Work out the finished part from the listing and answer in its coordinate system (mm). Face numbers are marked on the shaded views. A direction names the side the tool comes from. Coordinates: 2 decimals unless noted, no trailing zeros. Order: outer loops, then holes, each group sorted by start corner. A loop starts at its lowest first (then second) coordinate and runs counter-clockwise, first axis right, second up. Notation, with made-up numbers: (73, -8) -> (87, -8) arc R21 cw to (87, -1) -> close; hole circle Ø9 at (33, 66). An arc over 180 degrees is marked (long way). Write item = value, one per line. Start each with the question number.
Q1. Straight lines are drawn through the part: L1, parallel to Y at x = -243.2, z = 60; L2, parallel to Y at x = -25, z = 9.1; L3, parallel to X at y = -5.75, z = 85.5. For each, find the intervals that lie inside material, in ascending order. Write a range as from..to.
Q2. The part is cut by section C-C, the plane z = 60. Determine the outline of the cut face in (x, y).
Q3. The part is cut by section B-B, the plane x = -233. Determine the outline of the cut face in (y, z).
Q4. The part is cut by section D-D, the plane x = -49. Determine the outline of the cut face in (y, z).
Q5. Which of the six approach directions +Z, -Z, +X, -X, +Y, -Y give full straight-line access (tool end or side, diameter ignored) to the marked faces 1 and 2?
Q6. The part is cut by section A-A, the plane z = 104.5. Determine the outline of the cut face in (x, y), plus the area to 3 significant figures.
Q7. Flat-ended cylindrical pins translate along their axes: pin 1 (10 mm diameter, centred on y = 3, z = 135, fed in from +X); pin 2 (8 mm diameter, centred on y = 7, z = 112.5, fed in from +X); pin 3 (12.5 mm diameter, centred on x = -78.5, y = -3, fed in from +Z); pin 4 (15 mm diameter, centred on y = 3.5, z = 94, fed in from -X). Find the tip coordinate at first contact, or state that the pin passes through.
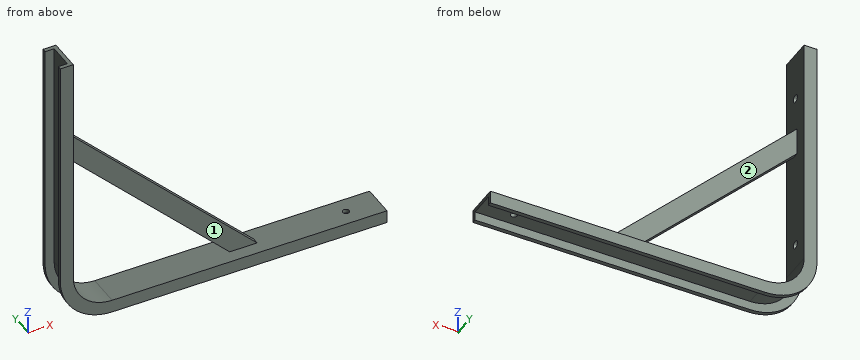
```python
from build123d import *

# Parameters (mm, degrees)
ESQUISSE1_W                  = 450
ESQUISSE1_H                  = 25
EXTRUSION1_DEPTH             = 10
PLIAGE_START                 = -12.5
PLIAGE_1_DEPTH               = 25
PLIAGE_1_2_DEPTH             = 25
ESQUISSE5_R                  = 3
ENL_V_MAT_EXTRU_1_DEPTH      = 330.361564282
ESQUISSE7_R                  = 2.5
ENL_V_MAT_EXTRU_2_DEPTH      = 331.27116136
ENL_V_MAT_EXTRU_3_DEPTH      = 9.5
ENL_V_MAT_EXTRU_3_DEPTH_BACK = 9.5
EXTRUSION2_DEPTH             = 2.5


# Read off the part's stored shape, not the designer's step: Pliage 1
with BuildPart() as part:
    # Esquisse1 → Extrusion1 (new body)
    with BuildSketch(Plane.XY):
        with Locations((-225, 0)):
            Rectangle(ESQUISSE1_W, ESQUISSE1_H)
    extrude(amount=EXTRUSION1_DEPTH)

    # Pliage 1 outline → Pliage 1 (cut)
    with BuildSketch(Plane(origin=(0, 0, 0), x_dir=(1, 0, 0), z_dir=(0, 1, 0)).offset(PLIAGE_START)):
        with BuildLine():
            Line((-450, -10), (-238.968577392, -10))
            ThreePointArc((-238.968577392, -10), (-226.653199905, -2.583426132), (-212.511064281, 0))
            Line((-212.511064281, 0), (-450, 0))
            Line((-450, 0), (-450, -10))
        make_face()
    extrude(amount=PLIAGE_1_DEPTH, mode=Mode.SUBTRACT)

    # Pliage 1 2 outline → Pliage 1 2 (add)
    with BuildSketch(Plane(origin=(0, 0, 0), x_dir=(1, 0, 0), z_dir=(0, 1, 0)).offset(PLIAGE_START)):
        with BuildLine():
            ThreePointArc((-238.968577392, -10), (-248.968577392, -23.542486889), (-252.511064281, -40))
            Line((-252.511064281, -40), (-252.511064281, -222.511064281))
            Line((-252.511064281, -222.511064281), (-242.511064281, -222.511064281))
            Line((-242.511064281, -222.511064281), (-242.511064281, -40))
            ThreePointArc((-242.511064281, -40), (-233.724267717, -18.786796564), (-212.511064281, -10))
            Line((-212.511064281, -10), (-238.968577392, -10))
        make_face()
    extrude(amount=PLIAGE_1_2_DEPTH)

    # Esquisse5 → Enlèv. mat.-Extru.1 (cut, through all)
    with BuildSketch(Plane(origin=(-242.511064281, 0, 0), x_dir=(0, 0, -1), z_dir=(1, 0, 0))):
        with Locations((-185, 0)):
            Circle(ESQUISSE5_R)
        with Locations((-60, 0)):
            Circle(ESQUISSE5_R)
    extrude(amount=-ENL_V_MAT_EXTRU_1_DEPTH, mode=Mode.SUBTRACT)

    # Esquisse7 → Enlèv. mat.-Extru.2 (cut, through all)
    with BuildSketch(Plane.XY.offset(10)):
        with Locations((-25, 0)):
            Circle(ESQUISSE7_R)
    extrude(amount=-ENL_V_MAT_EXTRU_2_DEPTH, mode=Mode.SUBTRACT)

    # Esquisse8 → Enlèv. mat.-Extru.3 (cut, two sides: drawn at the far end of the back side and taken through both)
    with BuildSketch(Plane(origin=(0, 0, 0), x_dir=(1, 0, 0), z_dir=(0, 1, 0)).offset(-ENL_V_MAT_EXTRU_3_DEPTH_BACK)):
        with BuildLine():
            Line((0, -7), (-212.511064281, -7))
            ThreePointArc((-212.511064281, -7), (-235.84558806, -16.665476221), (-245.511064281, -40))
            Line((-245.511064281, -40), (-245.511064281, -222.511064281))
            Line((-245.511064281, -222.511064281), (-252.511064281, -222.511064281))
            Line((-252.511064281, -222.511064281), (-252.511064281, -40))
            ThreePointArc((-252.511064281, -40), (-240.795335529, -11.715728753), (-212.511064281, 0))
            Line((-212.511064281, 0), (0, 0))
            Line((0, 0), (0, -7))
        make_face()
    extrude(amount=ENL_V_MAT_EXTRU_3_DEPTH + ENL_V_MAT_EXTRU_3_DEPTH_BACK, mode=Mode.SUBTRACT)

    # Esquisse6 → Extrusion2 (add, symmetric)
    with BuildSketch(Plane(origin=(0, 0, 0), x_dir=(1, 0, 0), z_dir=(0, 1, 0))):
        Polygon((-242.511064281, -136.297860845), (-116.213203436, -10), (-95, -10), (-242.511064281, -157.511064281), align=None)
    extrude(amount=EXTRUSION2_DEPTH, both=True)


solid = part.part
```
Model answer:
q1.L1 = -12.5..-3, 3..12.5
q1.L2 = -12.5..-2.5, 2.5..12.5
q1.L3 = -245.51..-242.51
q2.outline = (-252.51, -12.5) -> (-242.51, -12.5) -> (-242.51, -3) -> (-245.51, -3) -> (-245.51, -9.5) -> (-252.51, -9.5) -> close; (-252.51, 9.5) -> (-245.51, 9.5) -> (-245.51, 3) -> (-242.51, 3) -> (-242.51, 12.5) -> (-252.51, 12.5) -> close; (-166.21, -2.5) -> (-145, -2.5) -> (-145, 2.5) -> (-166.21, 2.5) -> close
q3.outline = (-12.5, 5.65) -> (-9.5, 5.65) -> (-9.5, 14.13) -> (9.5, 14.13) -> (9.5, 5.65) -> (12.5, 5.65) -> (12.5, 18.09) -> (-12.5, 18.09) -> close; (-2.5, 126.79) -> (2.5, 126.79) -> (2.5, 148) -> (-2.5, 148) -> close
q4.outline = (-12.5, 0) -> (-9.5, 0) -> (-9.5, 7) -> (9.5, 7) -> (9.5, 0) -> (12.5, 0) -> (12.5, 10) -> (-12.5, 10) -> close
q5.face_1 = +Z, +X, -Y
q5.face_2 = +Z, +X, +Y
q6.outline = (-252.51, -12.5) -> (-242.51, -12.5) -> (-242.51, 12.5) -> (-252.51, 12.5) -> (-252.51, 9.5) -> (-245.51, 9.5) -> (-245.51, -9.5) -> (-252.51, -9.5) -> close; (-210.71, -2.5) -> (-189.5, -2.5) -> (-189.5, 2.5) -> (-210.71, 2.5) -> close
q6.area = 223 mm2
q7.pin_1 = -215.03
q7.pin_2 = -242.51
q7.pin_3 = 10
q7.pin_4 = -252.51
